Verification items for this drawing (mm, ordinates from the low corner). A direction names the side the tool comes from. Coordinates: 2 decimals unless noted, no trailing zeros. Loops run counter-clockwise (first coordinate to the right, second up) from the corner with the lowest first, then second, coordinate; pieces in that order, holes last. Notation, with made-up numbers: M 8.5,87.5 L 52.5,87.5 A29 ccw 52.5,119.5 Z; hole C 74.25,38 d6. An arc over 180 degrees is marked long. One line per question, with ' | ' between items. Start each with the question number.
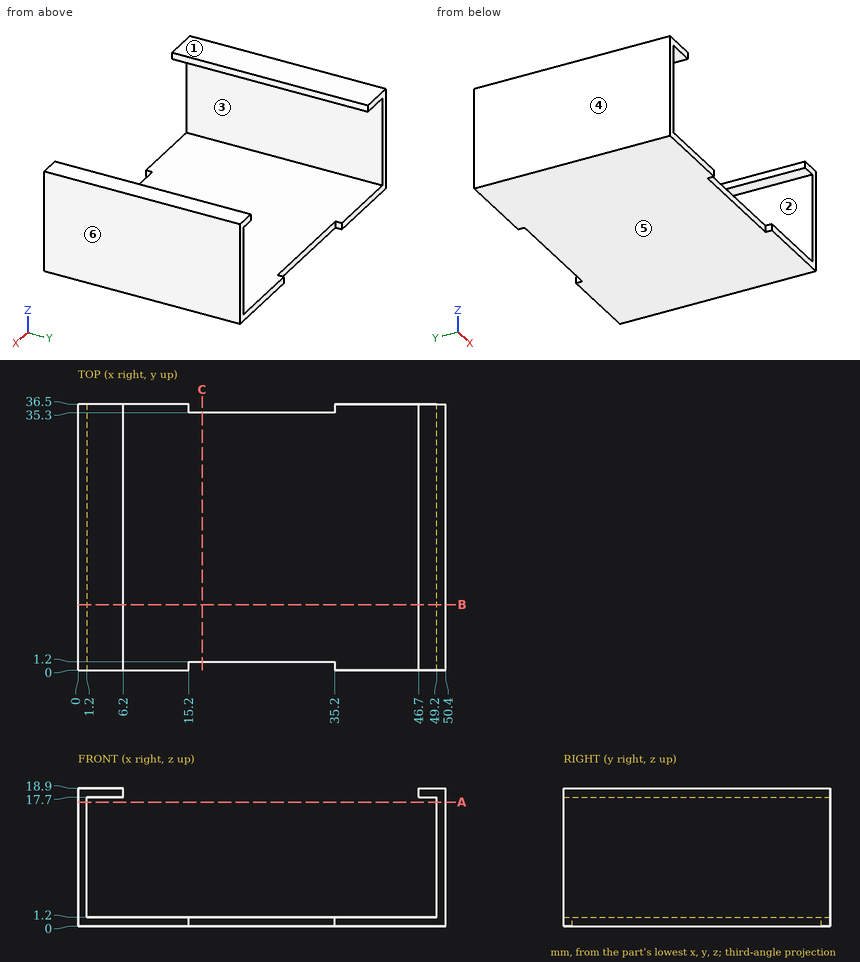
1. Sectioned sample at B-B (y = 9). Record the cut outline in (x, z), and give its area (3 significant figures).
2. Thickness scan on line 1 (X direction, y = 9, z = 8.75); line 2 (Z direction, x = 36, y = 4.5). Record the ranges inside material, lowest first.
3. Depth check by flat-ended pin: pin 1 Ø1.2 at (x, y) = (48.5, 18) entering from -Z; pin 2 Ø18 at (x, y) = (34, 23) entering from +Z; pin 3 Ø0.6 at (x, z) = (25.5, 0.5) entering from +Y; pin 4 Ø1.3 at (x, z) = (25.5, 0.5) entering from -Y. Enter the tip coordinate at first touch or a pass-through.
4. Draft check along X on the marked faces 3, 4, 5 and 6. Enter one of: +X half, -X half, draft (parallel to the pull), parting line (faces both ways), or undercut.
5. Sectioned sample at C-C (x = 17). Record the cut outline in (y, z).
6. Tool access check on the marked faces 1 and 2. Record the directions out of +Z, -Z, +X, -X, +Y, -Y that give a thin tool (end or side, any length) a straight path to the whole face; none if there is none.
7. Sectioned sample at A-A (z = 17). Record the cut outline in (x, y).
Result:
1) outline: M 0,0 L 50.4,0 L 50.4,18.9 L 46.7,18.9 L 46.7,17.7 L 49.2,17.7 L 49.2,1.2 L 1.2,1.2 L 1.2,17.7 L 6.2,17.7 L 6.2,18.9 L 0,18.9 Z | area: 112 mm2
2) line 1: x = 0 to 1.2, 49.2 to 50.4 | line 2: z = 0 to 1.2
3) pin 1: stops at z = 0 | pin 2: stops at z = 1.2 | pin 3: stops at y = 35.3 | pin 4: stops at y = 1.2
4) face 3: undercut | face 4: -X half | face 5: draft | face 6: +X half
5) outline: M 1.2,0 L 35.3,0 L 35.3,1.2 L 1.2,1.2 Z
6) face 1: +Z, +X, -X, +Y, -Y | face 2: +Y, -Y
7) outline: M 0,0 L 1.2,0 L 1.2,36.5 L 0,36.5 Z; M 49.2,0 L 50.4,0 L 50.4,36.5 L 49.2,36.5 Z
